For this review, take the finished solid that the model builds, in its own axes (mm). Face numbers are marked on the shaded views. A direction names the side the tool comes from. Round coordinates to 2 decimals unless told otherwise and drop trailing zeros. Order: outer loops, then holes, each group sorted by start corner. A loop starts at its lowest first (then second) coordinate and runs counter-clockwise, first axis right, second up. Notation, with made-up numbers: M 74.25,10.5 L 98.25,10.5 A23 ccw 98.25,19.5 Z; hole C -6,57 d11. An arc over 180 degrees is marked long. Answer as a JSON object with one key per item and string values.
from build123d import *

# Parameters (mm, degrees)
F0_W      = 28
F0_H      = 48
F1_DEPTH  = 25
F2_W      = 20
F2_H      = 37
F3_DEPTH  = 16
F4_R      = 3
F4_R_2    = 1.575
F5_DEPTH  = 2
F6_R      = 5
F6_R_2    = 3
F7_DEPTH  = 4
F8_R      = 4.25
F9_DEPTH  = 3
F10_DEPTH = 9.001
F14_DEPTH = 1
F17_DEPTH = 1
F18_R     = 1.74999


# Not quite as in the source:
# - a fillet or chamfer is up to 0.001 mm smaller than in the source, because OpenCascade refuses the exact size


with BuildPart() as f1:
    # F0 (on Top) → F1 (new body)
    with BuildSketch(Plane.XY):
        with Locations((-14, 24)):
            Rectangle(F0_W, F0_H)
    extrude(amount=F1_DEPTH)

    # F2 (on face) → F3 (cut)
    with BuildSketch(Plane.XY.offset(25)):
        with Locations((-14, 24)):
            Rectangle(F2_W, F2_H)
    extrude(amount=-F3_DEPTH, mode=Mode.SUBTRACT)

    # F4 (on face) → F5 (join)
    with BuildSketch(Plane.XY.offset(9)):
        with Locations((-11, 24)):
            Circle(F4_R)
        with Locations((-11, 24)):
            Circle(F4_R_2, mode=Mode.SUBTRACT)
    extrude(amount=F5_DEPTH)

    # F6 (on face) → F7 (cut)
    with BuildSketch(Plane.XY.offset(9)):
        with Locations((-11, 24)):
            Circle(F6_R)
        with Locations((-11, 24)):
            Circle(F6_R_2, mode=Mode.SUBTRACT)
    extrude(amount=-F7_DEPTH, mode=Mode.SUBTRACT)

    # F8 (on face) → F9 (cut)
    with BuildSketch(Plane(origin=(0, 5.5, 0), x_dir=(-1, 0, 0), z_dir=(0, 1, 0))):
        with Locations((18, 15)):
            Circle(F8_R)
    extrude(amount=-F9_DEPTH, mode=Mode.SUBTRACT)

    # F10 (cut, through all): a face of the model
    f10_faces = [f1.faces().sort_by_distance(p)[0] for p in [
        (-11, 24, 9),
    ]]
    extrude(f10_faces, amount=-F10_DEPTH, mode=Mode.SUBTRACT)

    # F13 (on face) → F14 (cut)
    with BuildSketch(Plane.XZ):
        with BuildLine():
            ThreePointArc((-19, 7.3008629454), (-18, 6.3008629454), (-17, 7.3008629454))
            Line((-17, 7.3008629454), (-17, 16.5))
            Line((-17, 16.5), (-17, 18.5))
            Line((-17, 18.5), (-18, 18.5))
            ThreePointArc((-18, 18.5), (-18.7071067812, 18.2071067812), (-19, 17.5))
            Line((-19, 17.5), (-19, 7.3008629454))
        make_face()
        with BuildLine():
            Line((-17, 18.5), (-17, 16.5))
            Line((-17, 16.5), (-11.7983063839, 16.5))
            ThreePointArc((-11.7983063839, 16.5), (-10.7983063839, 15.5), (-11.7983063839, 14.5))
            Line((-11.7983063839, 14.5), (-15, 14.5))
            ThreePointArc((-15, 14.5), (-14.5773817383, 14.406307787), (-14.2339555569, 14.1427876097))
            Line((-14.2339555569, 14.1427876097), (-12.8554930795, 12.5))
            Line((-12.8554930795, 12.5), (-11.7983063839, 12.5))
            ThreePointArc((-11.7983063839, 12.5), (-8.7983063839, 15.5), (-11.7983063839, 18.5))
            Line((-11.7983063839, 18.5), (-17, 18.5))
        make_face()
        with BuildLine():
            ThreePointArc((-14.2339555569, 14.1427876097), (-14.5773817383, 14.406307787), (-15, 14.5))
            ThreePointArc((-15, 14.5), (-15.906307787, 13.9226182617), (-15.7660444431, 12.8572123903))
            ThreePointArc((-15.7660444431, 12.8572123903), (-15.4226182617, 12.593692213), (-15, 12.5))
            ThreePointArc((-15, 12.5), (-14.2928932188, 12.7928932188), (-14, 13.5))
            ThreePointArc((-14, 13.5), (-14.0603073792, 13.8420201433), (-14.2339555569, 14.1427876097))
        make_face()
        with BuildLine():
            Line((-9.0322619408, 7.9436505551), (-12.8554930795, 12.5))
            Line((-12.8554930795, 12.5), (-15, 12.5))
            ThreePointArc((-15, 12.5), (-15.4226182617, 12.593692213), (-15.7660444431, 12.8572123903))
            Line((-15.7660444431, 12.8572123903), (-10.564350827, 6.6580753357))
            ThreePointArc((-10.564350827, 6.6580753357), (-9.1555187742, 6.5348185023), (-9.0322619408, 7.9436505551))
        make_face()
        with BuildLine():
            Line((-15, 12.5), (-12.8554930795, 12.5))
            Line((-12.8554930795, 12.5), (-14.2339555569, 14.1427876097))
            ThreePointArc((-14.2339555569, 14.1427876097), (-14.0603073792, 13.8420201433), (-14, 13.5))
            ThreePointArc((-14, 13.5), (-14.2928932188, 12.7928932188), (-15, 12.5))
        make_face()
    extrude(amount=-F14_DEPTH, mode=Mode.SUBTRACT)

    # F16 (on face) → F17 (cut)
    with BuildSketch(Plane(origin=(0, 5.5, 0), x_dir=(-1, 0, 0), z_dir=(0, 1, 0))):
        Polygon((9, 14.0925227119), (13.25, 16.5462613559), (13.25, 21.4537386441), (9, 23.9074772881), (4.75, 21.4537386441), (4.75, 16.5462613559), align=None)
        Polygon((9, 14.9585481157), (5.5, 16.9792740578), (5.5, 21.0207259422), (9, 23.0414518843), (12.5, 21.0207259422), (12.5, 16.9792740578), align=None, mode=Mode.SUBTRACT)
        with BuildLine():
            Line((7.5029805213, 17.2914120527), (6.6159696882, 17.7531606659))
            ThreePointArc((6.6159696882, 17.7531606659), (6.8286007981, 17.0787809427), (7.5029805213, 17.2914120527))
        make_face()
        with BuildLine():
            ThreePointArc((8.5564945834, 21.0191256934), (8.5, 21.25), (8.5564945834, 21.4808743066))
            Line((8.5564945834, 21.4808743066), (6.6159696882, 17.7531606659))
            Line((6.6159696882, 17.7531606659), (7.5029805213, 17.2914120527))
            Line((7.5029805213, 17.2914120527), (9, 20.1671597149))
            Line((9, 20.1671597149), (8.5564945834, 21.0191256934))
        make_face()
        with BuildLine():
            Line((9, 20.1671597149), (9.4435054166, 21.0191256934))
            ThreePointArc((9.4435054166, 21.0191256934), (9, 20.75), (8.5564945834, 21.0191256934))
            Line((8.5564945834, 21.0191256934), (9, 20.1671597149))
        make_face()
        with BuildLine():
            ThreePointArc((9.4435054166, 21.0191256934), (9.4856710349, 21.1311570538), (9.5, 21.25))
            ThreePointArc((9.5, 21.25), (9.4856710349, 21.3688429462), (9.4435054166, 21.4808743066))
            ThreePointArc((9.4435054166, 21.4808743066), (9, 21.75), (8.5564945834, 21.4808743066))
            ThreePointArc((8.5564945834, 21.4808743066), (8.5, 21.25), (8.5564945834, 21.0191256934))
            ThreePointArc((8.5564945834, 21.0191256934), (9, 20.75), (9.4435054166, 21.0191256934))
        make_face()
        with BuildLine():
            ThreePointArc((9.4435054166, 21.4808743066), (9.4856710349, 21.3688429462), (9.5, 21.25))
            ThreePointArc((9.5, 21.25), (9.4856710349, 21.1311570538), (9.4435054166, 21.0191256934))
            Line((9.4435054166, 21.0191256934), (9, 20.1671597149))
            Line((9, 20.1671597149), (10.4970194787, 17.2914120527))
            Line((10.4970194787, 17.2914120527), (11.3840303118, 17.7531606659))
            Line((11.3840303118, 17.7531606659), (9.4435054166, 21.4808743066))
        make_face()
        with BuildLine():
            ThreePointArc((10.4970194787, 17.2914120527), (11.1713992019, 17.0787809427), (11.3840303118, 17.7531606659))
            Line((11.3840303118, 17.7531606659), (10.4970194787, 17.2914120527))
        make_face()
    extrude(amount=-F17_DEPTH, mode=Mode.SUBTRACT)

    # F18 (radius 1.75 in the source; OpenCascade refuses exactly that, so slightly less here)
    f18_edges = [f1.edges().sort_by_distance(p)[0] for p in [
        (-24, 24, 9),
        (-14, 42.5, 9),
        (-4, 24, 9),
        (-14, 5.5, 9),
    ]]
    fillet(f18_edges, radius=F18_R)


solid = f1.part
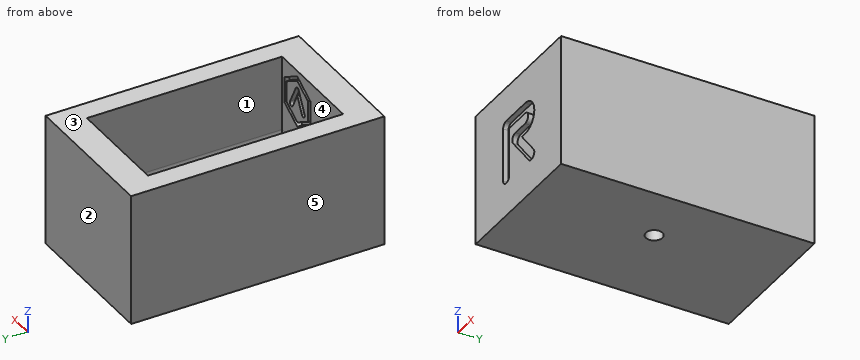
1) Add section D-D on z = 15.5. State the section outline as (x, y) points.
Geometry check:
{"outline": "M -28,0 L -19,0 L -19,1 L -17,1 L -17,0 L -10.8,0 L -10.8,1 L -8.8,1 L -8.8,0 L 0,0 L 0,48 L -28,48 Z; hole M -24,5.5 L -22.22,5.5 L -22.22,2.5 L -13.78,2.5 L -13.78,5.5 L -11.44,5.5 L -11.44,4.5 L -9.94,4.5 L -9.94,5.5 L -8.06,5.5 L -8.06,4.5 L -6.56,4.5 L -6.56,5.5 L -4,5.5 L -4,42.5 L -24,42.5 Z"}
2) Insertion check: P1, Ø4, axis at y = 19, z = 14.5, coming from the +X side; P2, Ø5, axis at x = -11, y = 24, coming from the +Z side. Each pin has a flat end and moves straight along its axis. Give the tip position at first contact, or say it passes through.
Geometry check:
{"P1": "stops at x = 0", "P2": "stops at z = 11"}
3) Machinability: for the marked faces 4 and 5, which of the approach directions +Z, -Z, +X, -X, +Y, -Y give a long, thin tool a straight path to every point of the face, cutting with its end or side? Answer none if there is none.
Geometry check:
{"face 4": "+Z", "face 5": "+Z, -Z, -X, +Y, -Y"}
4) For L1, parallel to Y at x = -20.5, z = 20.25; L2, parallel to Y at x = -11, z = 4.5 (3 decimals); L3, parallel to Y at x = -9.75, z = 8, list the stretches that pass through material, from the lowest coordinate up.
Geometry check:
{"L1": "y = 0 to 5.5, 42.5 to 48", "L2": "y = 0 to 22.425, 25.575 to 48", "L3": "y = 1 to 19.16, 21.27 to 23.04, 24.96 to 26.73, 28.84 to 48"}
5) Add section C-C on y = 31.5. State the section outline as (x, z) points.
Geometry check:
{"outline": "M -28,0 L 0,0 L 0,25 L -4,25 L -4,10.75 A1.75 cw -5.75,9 L -22.25,9 A1.75 cw -24,10.75 L -24,25 L -28,25 Z"}
6) Add section A-A on z = 5.5. State the section outline as (x, y) points (3 decimals), and give its area (3 significant figures).
Geometry check:
{"outline": "M -28,0 L 0,0 L 0,48 L -28,48 Z; C -11,24 d6; hole C -11,24 d10; hole C -11,24 d3.15", "area": "1,290 mm²"}
7) Add section B-B on y = 24. State the section outline as (x, z) points (3 decimals), and give its area (3 significant figures).
Geometry check:
{"outline": "M -28,0 L -12.575,0 L -12.575,11 L -14,11 L -14,5 L -16,5 L -16,9 L -22.25,9 A1.75 cw -24,10.75 L -24,25 L -28,25 Z; M -9.425,0 L 0,0 L 0,25 L -4,25 L -4,10.75 A1.75 cw -5.75,9 L -6,9 L -6,5 L -8,5 L -8,11 L -9.425,11 Z", "area": "343 mm²"}
8) Mouldability with a two-part tool opening along Y and no side actions: class the marked faces 1, 2 and 3 as +Y half, -Y half, draft (parallel to the pull), parting line (faces both ways), or undercut.
Geometry check:
{"face 1": "undercut", "face 2": "+Y half", "face 3": "draft"}
